from build123d import *

# Parameters (mm, degrees)
BOSS_EXTRUDE1_DEPTH = 2.5
SKETCH2_R           = 25
BOSS_EXTRUDE2_DEPTH = 5
SKETCH3_R           = 5
BOSS_EXTRUDE3_DEPTH = 25
SKETCH4_R           = 25
BOSS_EXTRUDE4_DEPTH = 5
SKETCH5_R           = 24.5
SKETCH5_R_2         = 5.5
BOSS_EXTRUDE5_DEPTH = 25


with BuildPart() as part:
    # Sketch1 → Boss-Extrude1 (new, symmetric)
    with BuildSketch(Plane.XY):
        Polygon((0, -125), (-108.253175473, 62.5), (108.253175473, 62.5), align=None)
        Polygon((0, -115), (-99.592921435, 57.5), (99.592921435, 57.5), align=None, mode=Mode.SUBTRACT)
    extrude(amount=BOSS_EXTRUDE1_DEPTH, both=True)

    # Sketch2 → Boss-Extrude2 (add)
    with BuildSketch(Plane.XY.offset(2.5)):
        with Locations((-108.253175473, 62.5)):
            Circle(SKETCH2_R)
        with Locations(Location((108.253175473, 62.5, 0), (0, 0, 180))):
            Circle(SKETCH2_R)
        with Locations(Location((0, -125, 0), (0, 0, 120))):
            Circle(SKETCH2_R)
    extrude(amount=BOSS_EXTRUDE2_DEPTH)

    # Sketch3 → Boss-Extrude3 (add)
    with BuildSketch(Plane.XY.offset(7.5)):
        with Locations((-108.253175473, 62.5)):
            Circle(SKETCH3_R)
        with Locations(Location((108.253175473, 62.5, 0), (0, 0, 180))):
            Circle(SKETCH3_R)
        with Locations((0, -125)):
            Circle(SKETCH3_R)
    extrude(amount=BOSS_EXTRUDE3_DEPTH)

    # Sketch4 → Boss-Extrude4 (add)
    with BuildSketch(Plane.XY.offset(32.5)):
        with Locations(Location((0, -125, 0), (0, 0, 120))):
            Circle(SKETCH4_R)
        with Locations(Location((108.253175473, 62.5, 0), (0, 0, 180))):
            Circle(SKETCH4_R)
        with Locations((-108.253175473, 62.5)):
            Circle(SKETCH4_R)
    extrude(amount=BOSS_EXTRUDE4_DEPTH)

    # Sketch5 → Boss-Extrude5 (add)
    # profile 1 of 3: a face of its own
    with BuildSketch(Plane.XY.offset(7.5)):
        with Locations((-108.253175473, 62.5)):
            Circle(SKETCH5_R)
        with Locations((-108.253175473, 62.5)):
            Circle(SKETCH5_R_2, mode=Mode.SUBTRACT)
    # profile 2 of 3: a face of its own
    with BuildSketch(Plane.XY.offset(7.5)):
        with Locations(Location((108.253175473, 62.5, 0), (0, 0, 180))):
            Circle(SKETCH5_R)
        with Locations((108.253175473, 62.5)):
            Circle(SKETCH5_R_2, mode=Mode.SUBTRACT)
    # profile 3 of 3: a face of its own
    with BuildSketch(Plane.XY.offset(7.5)):
        with Locations((0, -125)):
            Circle(SKETCH5_R)
        with Locations((0, -125)):
            Circle(SKETCH5_R_2, mode=Mode.SUBTRACT)
    extrude(amount=BOSS_EXTRUDE5_DEPTH)


solid = part.part
Could you check a few things on this model? Use its own coordinates, in mm. A direction names the side the tool comes from. Coordinates: 2 decimals unless noted, no trailing zeros. Write each loop counter-clockwise with the first axis right and the second up, starting at its lowest first coordinate (ties: lowest second). Pieces come first, ordered by that corner, then holes. Notation, with made-up numbers: M -10,26 L 49,26 A20 ccw 49,51 Z; hole C 47.5,44.25 d5. An arc over 180 degrees is marked long. One line per question, with ' | ' between items.
1) Imagine slicing it at D-D, the plane y = -136. Write out the boundary of the cut face in (x, z), and give its area (3 significant figures).
Checks:
outline: M -22.45,2.5 L 22.45,2.5 L 22.45,7.5 L 21.89,7.5 L 21.89,32.5 L 22.45,32.5 L 22.45,37.5 L -22.45,37.5 L -22.45,32.5 L -21.89,32.5 L -21.89,7.5 L -22.45,7.5 Z | area: 1,540 mm²
2) Imagine slicing it at B-B, the plane x = 28.5. Write out the boundary of the cut face in (y, z), and give its area (3 significant figures).
Checks:
outline: M -75.64,-2.5 L -65.64,-2.5 L -65.64,2.5 L -75.64,2.5 Z; M 57.5,-2.5 L 62.5,-2.5 L 62.5,2.5 L 57.5,2.5 Z | area: 75.0 mm²
3) If we mould it in two halves opening along X, with no side actions, what happens to faces 4 (the face through (-109, 63, 37.5)), 5 (the face through (54.884, -29.938, 0.035)), 6 (the face through (-3.19, -100.71, 19.82)), 7 (the face through (-111, 58, 32.5))? For each: released by +X, released by -X, zero draft, split by the parting line, or undercut.
Checks:
face 4: zero draft | face 5: released by +X | face 6: split by the parting line | face 7: undercut
4) Imagine slicing it at C-C, the plane y = -2.5. Write out the boundary of the cut face in (x, z).
Checks:
outline: M -70.73,-2.5 L -64.95,-2.5 L -64.95,2.5 L -70.73,2.5 Z; M 64.95,-2.5 L 70.73,-2.5 L 70.73,2.5 L 64.95,2.5 Z
5) For pin 1 Ø6 at (y, z) = (-4.5, 3) entering from -X; pin 2 Ø7 at (x, y) = (-89, 48) entering from -Z; pin 3 Ø3 at (x, z) = (-100.5, 18.5) entering from -Y; pin 4 Ø2 at (x, y) = (52, 56) entering from -Z, each with a flat end and sliding along its axis, tell me the tip position at first contact or that it passes through.
Checks:
pin 1: x = -71.28 | pin 2: z = 2.5 | pin 3: y = 38.81 | pin 4: through
6) For faces 1 (the face through (-0.1, -125.5, 2.5)), 2 (the face through (-91.7, 44.1, 7.5)), 3 (the face through (92, 52, 2.5)), which set-ups out of +Z, -Z, +X, -X, +Y, -Y let a thin tool reach every point of the face, with its end or its side?
Checks:
face 1: -Z, -Y | face 2: none | face 3: -Z
7) I need wall thicknesses on probe 1 along Y at (x, z) = (0, 18.25); probe 2 along Z at (x, y) = (-48, -35); probe 3 along Z at (x, y) = (118, 53). Which ranges of each line are inside material? Lowest first, please. Write a range as [from, to].
Checks:
probe 1: [-149.5, -130.5], [-130, -120], [-119.5, -100.5] | probe 2: [-2.5, 2.5] | probe 3: [2.5, 37.5]
8) Imagine slicing it at A-A, the plane z = 15. Give the number of separate pieces and of enclosed holes in the cut face, and give its area (3 significant figures).
Checks:
separate pieces: 6 | enclosed holes: 3 | area: 5,610 mm²
